Print and shaded views of the part. All mm, measured from the part's lowest x, y and z. A direction names the side the tool comes from. Round coordinates to 2 decimals unless told otherwise and drop trailing zeros. Loops run counter-clockwise (first coordinate to the right, second up) from the corner with the lowest first, then second, coordinate; pieces in that order, holes last. Notation, with made-up numbers: (48.5, 57) -> (103.5, 57) arc R26 cw to (103.5, 75) -> close; hole circle Ø2 at (7.5, 61.5). An arc over 180 degrees is marked (long way). Answer as CSV lines item,"result".
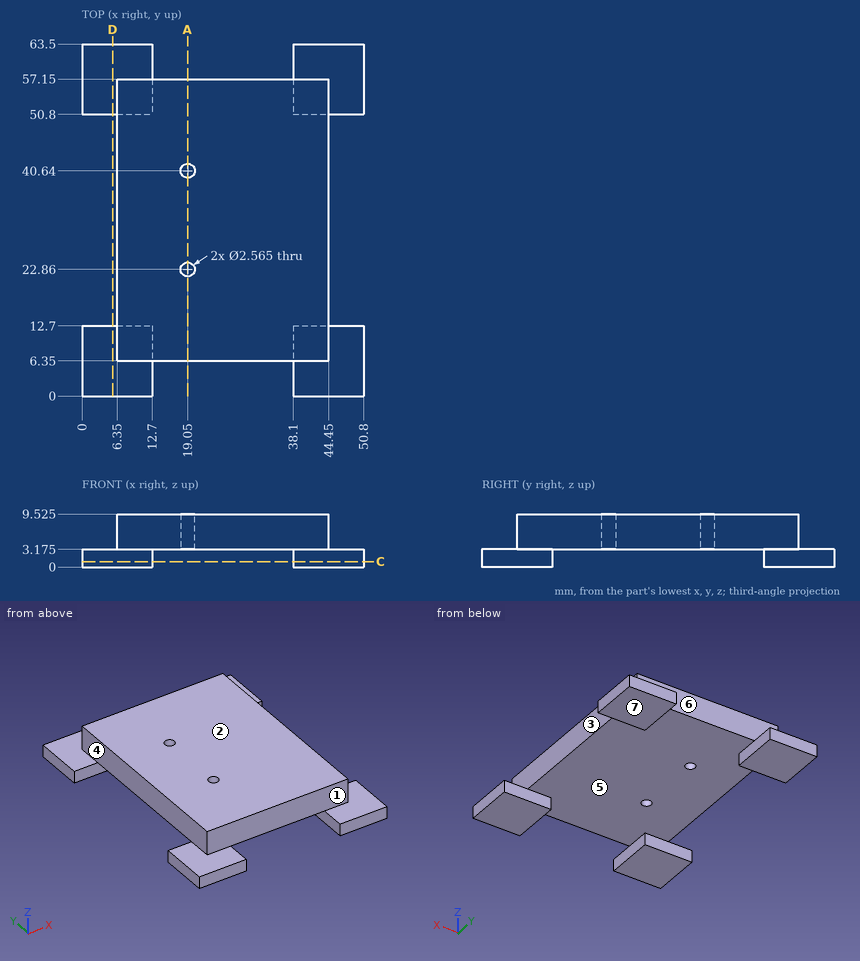
Q1. Saw through at D-D, the plane x = 5.5. Write the cut outline in (y, z) (1 decimal).
Geometry results:
outline,"(0, 0) -> (12.7, 0) -> (12.7, 3.2) -> (0, 3.2) -> close; (50.8, 0) -> (63.5, 0) -> (63.5, 3.2) -> (50.8, 3.2) -> close"
Q2. Saw through at C-C, the plane z = 1. Write the cut outline in (x, y), then the cut area to 3 significant figures.
Geometry results:
outline,"(0, 0) -> (12.7, 0) -> (12.7, 12.7) -> (0, 12.7) -> close; (0, 50.8) -> (12.7, 50.8) -> (12.7, 63.5) -> (0, 63.5) -> close; (38.1, 0) -> (50.8, 0) -> (50.8, 12.7) -> (38.1, 12.7) -> close; (38.1, 50.8) -> (50.8, 50.8) -> (50.8, 63.5) -> (38.1, 63.5) -> close"
area,"645 mm2"
Q3. Drop flat-ended pins along their axis: P1, Ø2.5, axis at x = 19.05, y = 40.64, coming from the +Z side; P2, Ø19, axis at x = 33, y = 25.5, coming from the -Z side (3 decimals); P3, Ø4, axis at x = 35, z = 6.5, coming from the +Y side; P4, Ø5, axis at y = 10.5, z = 8, coming from the +X side. Give the stop position or say it passes through.
Geometry results:
P1,"through"
P2,"z = 3.175"
P3,"y = 57.15"
P4,"x = 44.45"
Q4. Two-plate mould, pull along Y, no slides. Class the marked faces 5, 6 and 7: pulls with the +Y half, pulls with the -Y half, needs draft (parallel to the pull), parting line crosses it, or undercut.
Geometry results:
face 5,"undercut"
face 6,"pulls with the +Y half"
face 7,"needs draft"
Q5. Drill centre lines: line 1 along Y through (x, z) = (19.05, 7.25); line 2 along X through (y, z) = (22.86, 5.25); line 3 along Y through (x, z) = (8, 1). Where is each one in solid material? Low to high.
Geometry results:
line 1,"6.35 to 21.58, 24.14 to 39.36, 41.92 to 57.15"
line 2,"6.35 to 17.77, 20.33 to 44.45"
line 3,"0 to 12.7, 50.8 to 63.5"
Q6. Saw through at A-A, the plane x = 19.05. Give the number of separate pieces and of enclosed holes in the cut face, then the cut area to 3 significant figures.
Geometry results:
separate pieces,"3"
enclosed holes,"0"
area,"290 mm2"
Q7. Which spindle directions (+Z, -Z, +X, -X, +Y, -Y) get a long thin tool onto all of the face, cutting with end or side? Do the marked faces 1, 2, 3 and 4. Say none if no direction does.
Geometry results:
face 1,"+Z, +X, -X, -Y"
face 2,"+Z, +X, -X, +Y, -Y"
face 3,"+Z, +X, +Y, -Y"
face 4,"+Z, -X, +Y, -Y"
